Could you check a few things on this model? Use its own coordinates, in mm. Coordinates: 2 decimals unless noted, no trailing zeros. Loops run counter-clockwise (first coordinate to the right, second up) from the corner with the lowest first, then second, coordinate; pieces in that order, holes last. Notation, with made-up numbers: (68, -30) - (95, -30) arc R24 ccw to (95, 2) - close; hole circle Ø6 at (14, 35). An arc over 180 degrees is marked (long way). Put each result on its own line as item: value. Start each with the question number.
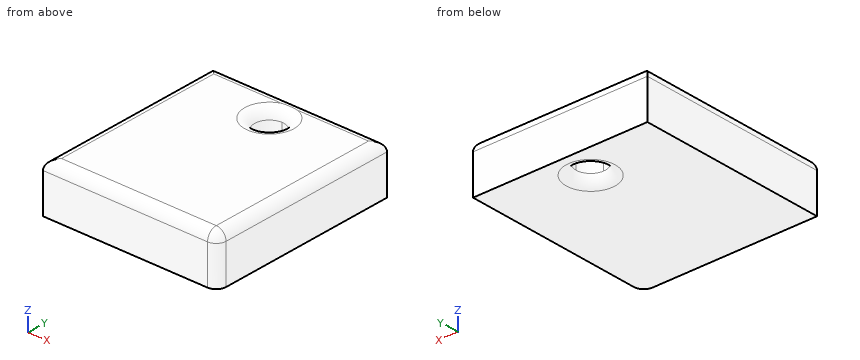
```python
from build123d import *

# Parameters (mm, degrees)
F1_DEPTH     = 25.4
F2_T1_DEPTH  = 97.6486100805
F2_T3_DEPTH  = 106.7304394197
F2_T5_DEPTH  = 33.02
F2_T7_DEPTH  = 115.4286100805
F2_T9_DEPTH  = 124.5104394197
F2_S13_W     = 5.08
F2_S13_H     = 5.08
F2_T14_DEPTH = 5.08


# Not quite as in the source:
# - a fillet or chamfer that OpenCascade refuses, or shapes differently, is made with other operations: its cross-section is extruded or revolved along the edge and cut away or added


with BuildPart() as f1:
    # F0 (on Top) → F1 (new body)
    with BuildSketch(Plane.XY):
        with BuildLine():
            Line((0, 51.6993701458), (-44.1247820854, 51.6993701458))
            Line((-44.1247820854, 51.6993701458), (-44.1247820854, -47.4110692739))
            Line((-44.1247820854, -47.4110692739), (0.8895229548, -47.4110692739))
            Line((0.8895229548, -47.4110692739), (0.8895229548, -45.8316206932))
            Line((0.8895229548, -45.8316206932), (0.223518183, 27.1919083226))
            ThreePointArc((0.223518183, 27.1919083226), (-7.3831209657, 34.6610501168), (0.0860208286, 42.2676892655))
            Line((0.0860208286, 42.2676892655), (0, 51.6993701458))
        make_face()
        with BuildLine():
            Line((45.9038279951, 51.6993701458), (0, 51.6993701458))
            Line((0, 51.6993701458), (0.0860208286, 42.2676892655))
            ThreePointArc((0.0860208286, 42.2676892655), (5.4607226524, 40.0843651019), (7.6929734789, 34.729798794))
            ThreePointArc((7.6929734789, 34.729798794), (5.5093358137, 29.4238456474), (0.223518183, 27.1919083226))
            Line((0.223518183, 27.1919083226), (0.8895229548, -45.8316206932))
            Line((0.8895229548, -45.8316206932), (0.8895229548, -47.4110692739))
            Line((0.8895229548, -47.4110692739), (45.9038279951, -47.4110692739))
            Line((45.9038279951, -47.4110692739), (45.9038279951, 51.6993701458))
        make_face()
    extrude(amount=F1_DEPTH)

    # F2: fillet of radius 5.08 on 8 edges, made by hand

    # F2_s2 → F2_t1 (cut)
    with BuildSketch(Plane.YZ.offset(-56.8247820854)):
        with BuildLine():
            ThreePointArc((-47.4110692739, 20.32), (-45.9231717224, 23.9121024484), (-42.3310692739, 25.4))
            Line((-42.3310692739, 25.4), (-47.4110692739, 25.4))
            Line((-47.4110692739, 25.4), (-47.4110692739, 20.32))
        make_face()
    extrude(amount=F2_T1_DEPTH, mode=Mode.SUBTRACT)

    # F2_s4 → F2_t3 (cut)
    with BuildSketch(Plane.XZ.offset(-64.3993701458)):
        with BuildLine():
            ThreePointArc((45.9038279951, 20.32), (44.4159304435, 23.9121024484), (40.8238279951, 25.4))
            Line((40.8238279951, 25.4), (45.9038279951, 25.4))
            Line((45.9038279951, 25.4), (45.9038279951, 20.32))
        make_face()
    extrude(amount=F2_T3_DEPTH, mode=Mode.SUBTRACT)

    # F2_s6 → F2_t5 (cut)
    with BuildSketch(Plane.XY.offset(-12.7)):
        with BuildLine():
            ThreePointArc((40.8238279951, -47.4110692739), (44.4159304435, -45.9231717224), (45.9038279951, -42.3310692739))
            Line((45.9038279951, -42.3310692739), (45.9038279951, -47.4110692739))
            Line((45.9038279951, -47.4110692739), (40.8238279951, -47.4110692739))
        make_face()
    extrude(amount=F2_T5_DEPTH, mode=Mode.SUBTRACT)

    # F2_s8 → F2_t7 (cut)
    with BuildSketch(Plane.YZ.offset(-56.8247820854)):
        with BuildLine():
            ThreePointArc((51.6993701458, 20.32), (50.2114725942, 23.9121024484), (46.6193701458, 25.4))
            Line((46.6193701458, 25.4), (51.6993701458, 25.4))
            Line((51.6993701458, 25.4), (51.6993701458, 20.32))
        make_face()
    extrude(amount=F2_T7_DEPTH, mode=Mode.SUBTRACT)

    # F2_s10 → F2_t9 (cut)
    with BuildSketch(Plane.XZ.offset(-64.3993701458)):
        with BuildLine():
            ThreePointArc((-44.1247820854, 20.32), (-42.6368845338, 23.9121024484), (-39.0447820854, 25.4))
            Line((-39.0447820854, 25.4), (-44.1247820854, 25.4))
            Line((-44.1247820854, 25.4), (-44.1247820854, 20.32))
        make_face()
    extrude(amount=F2_T9_DEPTH, mode=Mode.SUBTRACT)


with BuildPart() as f2_tool12:
    # F2_s13 → F2_t14 (new body)
    with BuildSketch(Plane.XZ.offset(42.3310692739)):
        with Locations((43.3638279951, 22.86)):
            Rectangle(F2_S13_W, F2_S13_H)
    extrude(amount=F2_T14_DEPTH)

    # F2_s15 → F2_t16 (revolve, cut)
    with BuildSketch(Plane(origin=(40.8238279951, -42.3310692739, 20.32), x_dir=(-0.7071067812, 0, -0.7071067812), z_dir=(-0.7071067812, 0, 0.7071067812))):
        with BuildLine():
            ThreePointArc((0, -5.08), (5.08, 0), (0, 5.08))
            Line((0, 5.08), (0, -5.08))
        make_face()
    revolve(axis=Axis((40.8238279951, -42.3310692739, 20.32), (0, -1, 0)), mode=Mode.SUBTRACT)


with BuildPart() as f1_1:
    add(f1.part)

    # F2_t11: cut F2_tool12
    add(f2_tool12.part, mode=Mode.SUBTRACT)

    # F2_s17 → F2_t18 (revolve, cut)
    with BuildSketch(Plane(origin=(0.4714804091, 0.0043000962, 0), x_dir=(0, 0, 1), z_dir=(-0.9999584116, -0.0091200341, 0))):
        with BuildLine():
            ThreePointArc((20.32, 42.265146908), (23.9121024484, 43.7530444596), (25.4, 47.345146908))
            Line((25.4, 47.345146908), (25.4, 42.265146908))
            Line((25.4, 42.265146908), (20.32, 42.265146908))
        make_face()
    revolve(axis=Axis((0.1547695058, 34.729798794, 25.4), (0, 0, -1)), mode=Mode.SUBTRACT)

    # F2_s19 → F2_t20 (revolve, cut)
    with BuildSketch(Plane(origin=(0.4714804091, 0.0043000962, 0), x_dir=(0, 0, 1), z_dir=(-0.9999584116, -0.0091200341, 0))):
        with BuildLine():
            ThreePointArc((5.08, 42.265146908), (1.4878975516, 43.7530444596), (0, 47.345146908))
            Line((0, 47.345146908), (0, 42.265146908))
            Line((0, 42.265146908), (5.08, 42.265146908))
        make_face()
    revolve(axis=Axis((0.1547695058, 34.729798794, 0), (0, 0, -1)), mode=Mode.SUBTRACT)


solid = f1_1.part
```
(1) For pin 1 Ø5 at (x, z) = (12.5, 22) entering from -Y, with a flat end and sliding along its axis, tell me the tip position at first contact or that it passes through.
(2) I need wall thicknesses on L1, parallel to X at y = -39.5, z = 20.75; L2, parallel to Y at x = 4, z = 21.5; L3, parallel to Y at x = -4.5, z = 23. Which ranges of each line are inside material? Lowest first, please. Write a range as [from, to].
(3) I want a section at A-A on z = 13.75. List the corners of the cut face in (x, y) for me.
(4) I want a section at B-B on z = 1.75. List the corners of the cut face in (x, y) for me, and give its area (3 significant figures).
Answer sheet:
1. pin 1: stops at y = -47.41
2. L1: x = [-44.11, 45.89]
2. L2: y = [-47.27, 28.09], [41.37, 51.56]
2. L3: y = [-46.65, 27.85], [41.6, 50.93]
3. outline: (-44.12, -47.41) - (40.82, -47.41) arc R5.08 ccw to (45.9, -42.33) - (45.9, 51.7) - (-44.12, 51.7) - close; hole circle Ø15.08 at (0.15, 34.73)
4. outline: (-44.12, -47.41) - (40.82, -47.41) arc R5.08 ccw to (45.9, -42.33) - (45.9, 51.7) - (-44.12, 51.7) - close; hole circle Ø17.56 at (0.15, 34.73)
4. area: 8,670 mm^2
